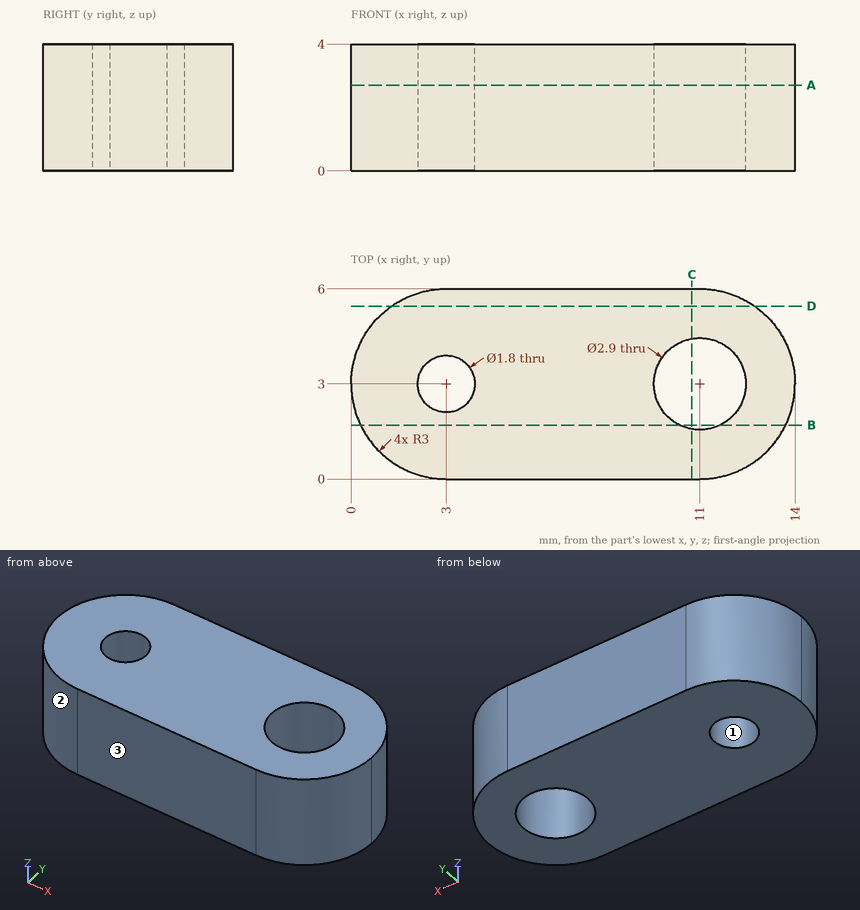
Print and shaded views of the part. All mm, measured from the part's lowest x, y and z. Coordinates: 2 decimals unless noted, no trailing zeros. Order: outer loops, then holes, each group sorted by start corner. A loop starts at its lowest first (then second) coordinate and runs counter-clockwise, first axis right, second up.
Item 1: Drop a flat-ended pin along its axis: pin 1 Ø2.5 at (x, y) = (11, 3) entering from +Z. Give the stop position or say it passes through.
Filled in:
pin 1: passes through
Item 2: Drill centre lines: L1, parallel to X at y = 3, z = 2.15; L2, parallel to Y at x = 11, z = 1.3; L3, parallel to Y at x = 3, z = 3. Where is each one in solid material? Low to high.
Filled in:
L1: x = 0 to 2.1, 3.9 to 9.55, 12.45 to 14
L2: y = 0 to 1.55, 4.45 to 6
L3: y = 0 to 2.1, 3.9 to 6
Item 3: Saw through at B-B on y = 1.7. List the corners of the cut face in (x, z), then the cut area to 3 significant figures.
Filled in:
outline: (0.3, 0) - (10.36, 0) - (10.36, 4) - (0.3, 4) - close; (11.64, 0) - (13.7, 0) - (13.7, 4) - (11.64, 4) - close
area: 48.5 mm2
Item 4: Saw through at A-A on z = 2.7. State how many separate pieces and enclosed holes the cut face has, then the cut area to 3 significant figures.
Filled in:
separate pieces: 1
enclosed holes: 2
area: 67.1 mm2
Item 5: Saw through at C-C on x = 10.75. List the corners of the cut face in (y, z), then the cut area to 3 significant figures.
Filled in:
outline: (0, 0) - (1.57, 0) - (1.57, 4) - (0, 4) - close; (4.43, 0) - (6, 0) - (6, 4) - (4.43, 4) - close
area: 12.6 mm2
Item 6: Saw through at D-D on y = 5.45. List the corners of the cut face in (x, z).
Filled in:
outline: (1.27, 0) - (12.73, 0) - (12.73, 4) - (1.27, 4) - close
Item 7: Mould opens along X. For the marked faces 1, 2 and 3 say: released by +X, released by -X, zero draft, split by the parting line, or undercut.
Filled in:
face 1: undercut
face 2: released by -X
face 3: zero draft
